For this review, use the dimensioned drawing (mm, ordinates from the lowest corner) and the shaded views. Round coordinates to 2 decimals unless told otherwise and drop trailing zeros. Loops run counter-clockwise (first coordinate to the right, second up) from the corner with the lowest first, then second, coordinate; pieces in that order, holes last. Notation, with made-up numbers: M 39.5,-15 L 80.5,-15 A11 ccw 80.5,-8 Z; hole C -14,15.25 d7. An arc over 180 degrees is marked long. One line per item, written item: value. Start each with the question number.
Item 1: Mouldability with a two-part tool opening along Z and no side actions: class the marked faces 1, 2, 3 and 4 as released by +Z, released by -Z, zero draft, split by the parting line, or undercut.
Item 2: We need section B-B (z = 275). Write out the cut boundary in (x, y).
Item 3: Clearance check with flat-ended pins moving along their axes: pin 1 (8 mm diameter, centred on x = 232.5, y = 179.5, fed in from +Z); pin 2 (12 mm diameter, centred on y = 52.5, z = 196.5, fed in from -X); pin 3 (2 mm diameter, centred on x = 72, z = 286.5, fed in from -Y); pin 4 (2 mm diameter, centred on y = 80.5, z = 333, fed in from -X). State where each tip first meets the part, or that it passes through.
Item 4: For line 1 along X through (y, z) = (13.95, 275); line 2 along X through (y, z) = (219.5, 233); line 3 along Y through (x, z) = (227, 193.5), list the stretches that pass through material, from the lowest coordinate up.
Item 5: We need section A-A (x = 275). Write out the cut boundary in (y, z), then the cut area to 3 significant figures.
Item 6: We need section C-C (y = 116). Write out the cut boundary in (x, z), then the cut area to 3 significant figures.
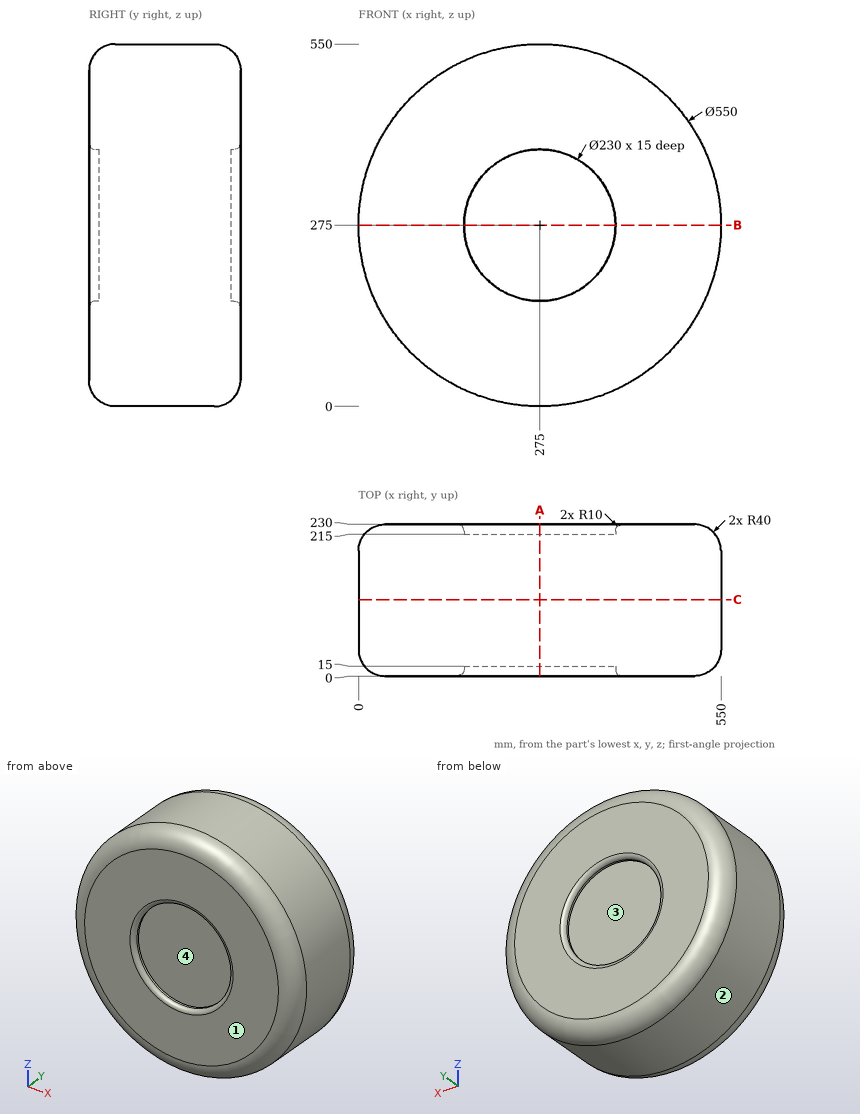
A:
1. face 1: zero draft
1. face 2: split by the parting line
1. face 3: undercut
1. face 4: undercut
2. outline: M 0,40 A40 ccw 40,0 L 150,0 A10 ccw 160,10 L 160,15 L 390,15 L 390,10 A10 ccw 400,0 L 510,0 A40 ccw 550,40 L 550,190 A40 ccw 510,230 L 400,230 A10 ccw 390,220 L 390,215 L 160,215 L 160,220 A10 ccw 150,230 L 40,230 A40 ccw 0,190 Z
3. pin 1: z = 547.29
3. pin 2: x = 9.73
3. pin 3: y = 0
3. pin 4: x = 5.97
4. line 1: 9.65 to 160, 390 to 540.35
4. line 2: 16.37 to 167.94, 382.06 to 533.63
4. line 3: 15 to 215
5. outline: M 0,40 A40 ccw 40,0 L 190,0 A40 ccw 230,40 L 230,150 A10 ccw 220,160 L 215,160 L 215,390 L 220,390 A10 ccw 230,400 L 230,510 A40 ccw 190,550 L 40,550 A40 ccw 0,510 L 0,400 A10 ccw 10,390 L 15,390 L 15,160 L 10,160 A10 ccw 0,150 Z
5. area: 118,000 mm2
6. outline: C 275,275 d550
6. area: 238,000 mm2
